Check sheet for the modelled part. Datum: model origin and axes. Units: mm. A direction names the side the tool comes from. Round coordinates to 2 decimals unless told otherwise and drop trailing zeros. Loops run counter-clockwise (first coordinate to the right, second up) from the corner with the lowest first, then second, coordinate; pieces in that order, holes last. Notation, with made-up numbers: M -6,15 L 48,15 A6 ccw 48,22 Z; hole C 0.5,34 d6. An arc over 180 degrees is marked long. Write item = value, one per line. Start each with the question number.
(1) Go/stop test with flat-tipped pins: P1, Ø12, axis at y = -60.5, z = 36.5, coming from the +X side; P2, Ø8, axis at x = -35.5, z = 13, coming from the -Y side; P3, Ø12, axis at y = -56.5, z = 24.5, coming from the +X side; P4, Ø4, axis at y = -22.5, z = 20, coming from the -X side. Record where each tip stops, or that it passes through.
(2) Scan lines: L1, parallel to Z at x = -40, y = -71; L2, parallel to X at y = -18.5, z = 34; L3, parallel to Z at x = -38.5, y = -50.5. Record each from-to range of solid material in increasing order. Write a range as from..to.
(3) Cross-section at C-C on x = -46. Record the boundary of the cut face in (y, z), plus the area to 3 significant figures.
(4) Mould release check, pull along X, two halves, no side actions. Record for faces 3 (the face through (-38.1, -45, 10)), 4 (the face through (-45, -44, 0)), 5 (the face through (-38.92, -37.57, 25.21)): pulls with the +X half, pulls with the -X half, needs draft (parallel to the pull), parting line crosses it, or undercut.
(5) Set-up check for faces 1 (the face through (-39, 0, 25)), 2 (the face through (-50.8, -45, 12)): record each of +Z, -Z, +X, -X, +Y, -Y from which the full face is reachable in a straight line by a thin tool's end or side.
(6) Cross-section at D-D on z = 7. Record the boundary of the cut face in (x, y).
(7) Cross-section at B-B on z = 33. Record the boundary of the cut face in (x, y), plus the area to 3 significant figures.
from build123d import *

# Parameters (mm, degrees)
F1_DEPTH = 76.2
F2_W     = 12.7
F2_H     = 12.7
F3_DEPTH = 23.622


with BuildPart() as f1:
    # F0 (on Front) → F1 (new body)
    with BuildSketch(Plane.XZ):
        with BuildLine():
            Line((-55.64358, 41.81907), (-60.72358, 41.81907))
            ThreePointArc((-60.72358, 41.81907), (-39.336659, 20.23352), (-17.949738, 41.81907))
            Line((-17.949738, 41.81907), (-22.914561, 41.81907))
            ThreePointArc((-22.914561, 41.81907), (-39.27907, 25.205913), (-55.64358, 41.81907))
        make_face()
    extrude(amount=F1_DEPTH)

    # F2 (on Top) → F3 (join)
    with BuildSketch(Plane.XY):
        with Locations((-44.45, -44.45)):
            Rectangle(F2_W, F2_H)
    extrude(amount=F3_DEPTH)


solid = f1.part
Result:
q1.P1 = -17.95
q1.P2 = -50.8
q1.P3 = -21.07
q1.P4 = -47.85
q2.L1 = 20.24..25.22
q2.L2 = -59.32..-53.79, -24.77..-19.35
q2.L3 = 0..25.22
q3.outline = M -76.2,21.3 L -50.8,21.3 L -50.8,0 L -38.1,0 L -38.1,21.3 L 0,21.3 L 0,26.65 L -76.2,26.65 Z
q3.area = 678 mm^2
q4.face_3 = pulls with the +X half
q4.face_4 = needs draft
q4.face_5 = undercut
q5.face_1 = +Z, -Z, +X, -X, +Y
q5.face_2 = -Z, -X, +Y, -Y
q6.outline = M -50.8,-50.8 L -38.1,-50.8 L -38.1,-38.1 L -50.8,-38.1 Z
q7.outline = M -58.91,-76.2 L -53.22,-76.2 L -53.22,0 L -58.91,0 Z; M -25.34,-76.2 L -19.76,-76.2 L -19.76,0 L -25.34,0 Z
q7.area = 858 mm^2
